Check sheet for the modelled part. Datum: model origin and axes. Units: mm. Coordinates: 2 decimals unless noted, no trailing zeros. Order: outer loops, then holes, each group sorted by start corner. A loop starts at its lowest first (then second) coordinate and runs counter-clockwise, first axis right, second up. Notation, with made-up numbers: (63.5, 53.25) -> (122.5, 53.25) arc R25 cw to (122.5, 66.25) -> close; hole circle Ø1 at (-24.5, 25.5). An arc over 180 degrees is marked (long way). Put each result on its own line as item: value. Start each with the question number.
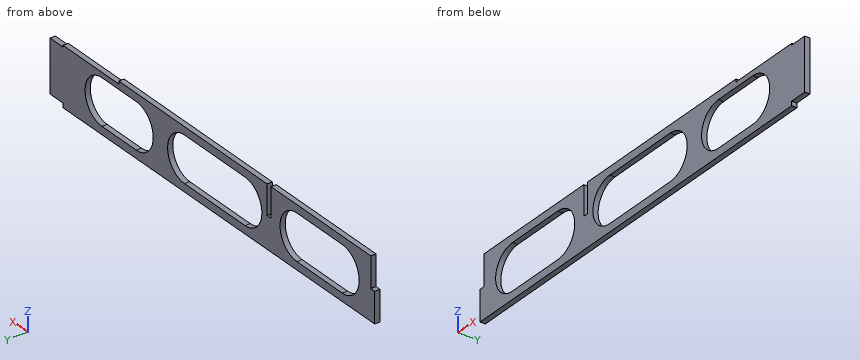
```python
from build123d import *

# Parameters (mm, degrees)
SKETCH1_W               = 250.28
SKETCH1_H               = 35
BOSS_EXTRUDE1_DEPTH     = 3
SKETCH2_W               = 3
SKETCH2_H               = 17
CUT_EXTRUDE1_DEPTH      = 1
CUT_EXTRUDE1_DEPTH_BACK = 4
CUT_EXTRUDE3_DEPTH      = 4
SKETCH5_W               = 10
SKETCH5_H               = 2.5
CUT_EXTRUDE4_DEPTH      = 3
SKETCH6_W               = 3
SKETCH6_H               = 17.5
CUT_EXTRUDE5_DEPTH      = 10
SKETCH7_W               = 43
SKETCH7_H               = 3
CUT_EXTRUDE6_DEPTH      = 1.6


with BuildPart() as part:
    # Sketch1 → Boss-Extrude1 (new body)
    with BuildSketch(Plane(origin=(0, 0, 0), x_dir=(1, 0, 0), z_dir=(0, 1, 0))):
        with Locations((125.14, 0)):
            Rectangle(SKETCH1_W, SKETCH1_H)
    extrude(amount=BOSS_EXTRUDE1_DEPTH)

    # Sketch2 → Cut-Extrude1 (cut, two sides)
    with BuildSketch(Plane(origin=(0, 3, 0), x_dir=(1, 0, 0), z_dir=(0, 1, 0))) as cut_extrude1_sk:
        with Locations((81.5, -9)):
            Rectangle(SKETCH2_W, SKETCH2_H)
    extrude(amount=CUT_EXTRUDE1_DEPTH, mode=Mode.SUBTRACT)
    extrude(cut_extrude1_sk.sketch, amount=-CUT_EXTRUDE1_DEPTH_BACK, mode=Mode.SUBTRACT)

    # Sketch4 → Cut-Extrude3 (cut, through all)
    with BuildSketch(Plane(origin=(0, 3, 0), x_dir=(1, 0, 0), z_dir=(0, 1, 0))):
        with BuildLine():
            Line((183.762367309, 13), (210.28, 13))
            ThreePointArc((210.28, 13), (223.28, 0), (210.28, -13))
            Line((210.28, -13), (183.762367309, -13))
            ThreePointArc((183.762367309, -13), (170.762367309, 0), (183.762367309, 13))
        make_face()
        with BuildLine():
            Line((25, 13), (60, 13))
            ThreePointArc((60, 13), (73, 0), (60, -13))
            Line((60, -13), (25, -13))
            ThreePointArc((25, -13), (12, 0), (25, 13))
        make_face()
        with BuildLine():
            Line((100, 13), (146.655192757, 13))
            ThreePointArc((146.655192757, 13), (159.655192757, 0), (146.655192757, -13))
            Line((146.655192757, -13), (100, -13))
            ThreePointArc((100, -13), (87, 0), (100, 13))
        make_face()
    extrude(amount=-CUT_EXTRUDE3_DEPTH, mode=Mode.SUBTRACT)

    # Sketch5 → Cut-Extrude4 (cut)
    with BuildSketch(Plane(origin=(0, 3, 0), x_dir=(1, 0, 0), z_dir=(0, 1, 0))):
        with Locations((245.28, 16.25)):
            Rectangle(SKETCH5_W, SKETCH5_H)
        with Locations((245.28, -16.25)):
            Rectangle(SKETCH5_W, SKETCH5_H)
    extrude(amount=-CUT_EXTRUDE4_DEPTH, mode=Mode.SUBTRACT)

    # Sketch6 → Cut-Extrude5 (cut)
    with BuildSketch(Plane(origin=(0, 3, 0), x_dir=(1, 0, 0), z_dir=(0, 1, 0))):
        with Locations((1.5, -8.75)):
            Rectangle(SKETCH6_W, SKETCH6_H)
    extrude(amount=-CUT_EXTRUDE5_DEPTH, mode=Mode.SUBTRACT)

    # Sketch7 → Cut-Extrude6 (cut)
    with BuildSketch(Plane.XY.offset(17.5)):
        with Locations((218.78, 1.5)):
            Rectangle(SKETCH7_W, SKETCH7_H)
    extrude(amount=-CUT_EXTRUDE6_DEPTH, mode=Mode.SUBTRACT)


solid = part.part
```
1) Sectioned sample at C-C (y = 2.05). Record the boundary of the cut face in (x, z).
2) Sectioned sample at D-D (z = 7). Record the boundary of the cut face in (x, y), plus the area to 3 significant figures.
3) Gauge pin test, flat ends, axial feed: pin 1 (0.9 mm diameter, centred on x = 1, y = 1.5, fed in from +Z); pin 2 (1.5 mm diameter, centred on x = 227, y = 2, fed in from +Z); pin 3 (1.3 mm diameter, centred on y = 2, z = 16.5, fed in from +X). Record the tip position at first contact, or that the pin passes through.
4) Scan lines: line 1 along X through (y, z) = (1.9, 1); line 2 along Z through (x, y) = (124, 1.6); line 3 along X through (y, z) = (1.5, 2.5). Record each from-to range of solid material in increasing order. Write a range as [from, to].
5) Sectioned sample at A-A (x = 131.5). Record the boundary of the cut face in (y, z).
6) Sectioned sample at B-B (z = -4.5). Record the boundary of the cut face in (x, y), plus the area to 3 significant figures.
Entries:
1. outline: (0, -17.5) -> (240.28, -17.5) -> (240.28, -15) -> (250.28, -15) -> (250.28, 15) -> (240.28, 15) -> (240.28, 15.9) -> (197.28, 15.9) -> (197.28, 17.5) -> (83, 17.5) -> (83, 0.5) -> (80, 0.5) -> (80, 17.5) -> (3, 17.5) -> (3, 0) -> (0, 0) -> close; hole (25, -13) -> (60, -13) arc R13 ccw to (60, 13) -> (25, 13) arc R13 ccw to start; hole (100, -13) -> (146.66, -13) arc R13 ccw to (146.66, 13) -> (100, 13) arc R13 ccw to start; hole (183.76, -13) -> (210.28, -13) arc R13 ccw to (210.28, 13) -> (183.76, 13) arc R13 ccw to start
2. outline: (3, 0) -> (14.05, 0) -> (14.05, 3) -> (3, 3) -> close; (70.95, 0) -> (80, 0) -> (80, 3) -> (70.95, 3) -> close; (83, 0) -> (89.05, 0) -> (89.05, 3) -> (83, 3) -> close; (157.61, 0) -> (172.81, 0) -> (172.81, 3) -> (157.61, 3) -> close; (221.23, 0) -> (250.28, 0) -> (250.28, 3) -> (221.23, 3) -> close
2. area: 211 mm2
3. pin 1: stops at z = 0
3. pin 2: stops at z = 15.9
3. pin 3: stops at x = 240.28
4. line 1: x = [3, 12.04], [72.96, 80], [83, 87.04], [159.62, 170.8], [223.24, 250.28]
4. line 2: z = [-17.5, -13], [13, 17.5]
4. line 3: x = [3, 12.24], [72.76, 80], [83, 87.24], [159.41, 171.01], [223.04, 250.28]
5. outline: (0, -17.5) -> (3, -17.5) -> (3, -13) -> (0, -13) -> close; (0, 13) -> (3, 13) -> (3, 17.5) -> (0, 17.5) -> close
6. outline: (0, 0) -> (12.8, 0) -> (12.8, 3) -> (0, 3) -> close; (72.2, 0) -> (87.8, 0) -> (87.8, 3) -> (72.2, 3) -> close; (158.85, 0) -> (171.57, 0) -> (171.57, 3) -> (158.85, 3) -> close; (222.48, 0) -> (250.28, 0) -> (250.28, 3) -> (222.48, 3) -> close
6. area: 207 mm2
